The listing builds one solid part. Answer for the finished solid, in the listing's coordinates (mm). Face numbers are marked on the shaded views. A direction names the side the tool comes from. Coordinates: 2 decimals unless noted, no trailing zeros. Order: outer loops, then holes, each group sorted by start corner. A loop starts at its lowest first (then second) coordinate and runs counter-clockwise, first axis right, second up. Notation, with made-up numbers: (-8, 66.25) -> (25, 66.25) arc R21 ccw to (25, 103.25) -> close; hole circle Ø6 at (70, -5). An arc over 180 degrees is marked (long way). Put each result on its own line as item: value. Start each with the question number.
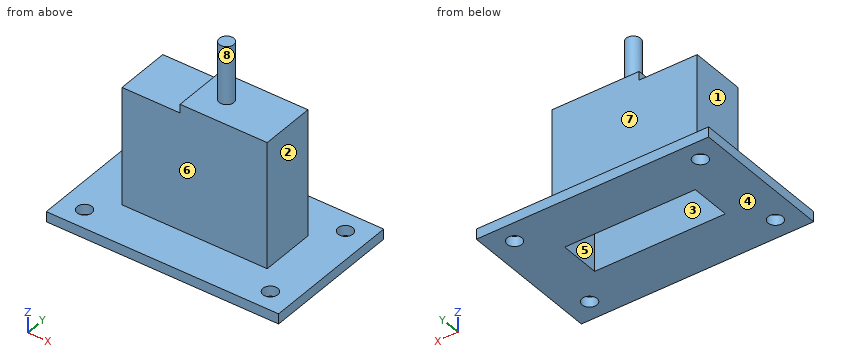
```python
from build123d import *

# Parameters (mm, degrees)
F0_W      = 50
F0_H      = 19
F1_DEPTH  = 44
F2_W      = 30
F2_H      = 19
F3_DEPTH  = 3
F4_R      = 2.5
F5_DEPTH  = 20
F6_W      = 80
F6_H      = 49
F7_DEPTH  = 3.5
F8_R      = 2.55
F9_DEPTH  = 3.5
F10_W     = 45
F10_H     = 14
F11_DEPTH = 42


with BuildPart() as f1:
    # F0 (on Top) → F1 (new body)
    with BuildSketch(Plane.XY):
        Rectangle(F0_W, F0_H)
    extrude(amount=F1_DEPTH)

    # F2 (on face) → F3 (join)
    with BuildSketch(Plane.XY.offset(44)):
        with Locations((10, 0)):
            Rectangle(F2_W, F2_H)
    extrude(amount=F3_DEPTH)

    # F4 (on face) → F5 (join)
    with BuildSketch(Plane.XY.offset(47)):
        with Locations((4, 0)):
            Circle(F4_R)
    extrude(amount=F5_DEPTH)

    # F6 (on face) → F7 (join)
    with BuildSketch(Plane(origin=(0, 0, 0), x_dir=(1, 0, 0), z_dir=(0, 0, -1))):
        Rectangle(F6_W, F6_H)
    extrude(amount=-F7_DEPTH)

    # F8 (on face) → F9 (cut, through all)
    with BuildSketch(Plane.XY.offset(3.5)):
        with Locations((-32, 17.5)):
            Circle(F8_R)
        with Locations((32, 17.5)):
            Circle(F8_R)
        with Locations((-32, -17.5)):
            Circle(F8_R)
        with Locations((32, -17.5)):
            Circle(F8_R)
    extrude(amount=-F9_DEPTH, mode=Mode.SUBTRACT)

    # F10 (on face) → F11 (cut)
    with BuildSketch(Plane(origin=(0, 0, 0), x_dir=(1, 0, 0), z_dir=(0, 0, -1))):
        Rectangle(F10_W, F10_H)
    extrude(amount=-F11_DEPTH, mode=Mode.SUBTRACT)


solid = f1.part
```
(1) Find the intervals of material crossed by L1, parallel to Y at x = 32, z = 1.15; L2, parallel to Y at x = 16, z = 29.5; L3, parallel to X at y = -2, z = 5, in increasing order.
(2) The part is cut by section B-B on z = 18. Determine the outline of the cut face in (x, y).
(3) The part is cut by section D-D on x = 4. Determine the outline of the cut face in (y, z).
(4) The part is cut by section C-C on x = -32. Determine the outline of the cut face in (y, z).
(5) Each of these flat-tipped pins is pushed along its axis until it touches: P1, Ø6, axis at x = -32, y = -17.5, coming from the +Z side; P2, Ø22, axis at x = 1.5, z = 33, coming from the +Y side; P3, Ø4, axis at x = 10, y = -1.5, coming from the -Z side; P4, Ø4, axis at x = 32, y = -17.5, coming from the -Z side. Where does it stop, or does it pass through?
(6) A tool of negligible diameter and unlimited length cuts with its end or side. For the marked faces 5, 6, 7 and 8, from which of +Z, -Z, +X, -X, +Y, -Y can it reach the whole face along a straight path? Write none if from no direction.
(7) For a pull along X with two mould halves and no side action, classify the marked faces 1, 2, 3 and 4 as released by +X, released by -X, zero draft, split by the parting line, or undercut.
(8) The part is cut by section A-A on y = -17.5. Determine the outline of the cut face in (x, z), plus the area to 3 significant figures.
Worked out:
1. L1: -24.5 to -20.05, -14.95 to 14.95, 20.05 to 24.5
1. L2: -9.5 to -7, 7 to 9.5
1. L3: -25 to -22.5, 22.5 to 25
2. outline: (-25, -9.5) -> (25, -9.5) -> (25, 9.5) -> (-25, 9.5) -> close; hole (-22.5, -7) -> (22.5, -7) -> (22.5, 7) -> (-22.5, 7) -> close
3. outline: (-24.5, 0) -> (-7, 0) -> (-7, 42) -> (7, 42) -> (7, 0) -> (24.5, 0) -> (24.5, 3.5) -> (9.5, 3.5) -> (9.5, 47) -> (2.5, 47) -> (2.5, 67) -> (-2.5, 67) -> (-2.5, 47) -> (-9.5, 47) -> (-9.5, 3.5) -> (-24.5, 3.5) -> close
4. outline: (-24.5, 0) -> (-20.05, 0) -> (-20.05, 3.5) -> (-24.5, 3.5) -> close; (-14.95, 0) -> (14.95, 0) -> (14.95, 3.5) -> (-14.95, 3.5) -> close; (20.05, 0) -> (24.5, 0) -> (24.5, 3.5) -> (20.05, 3.5) -> close
5. P1: z = 3.5
5. P2: y = 9.5
5. P3: z = 42
5. P4: through
6. face 5: -Z
6. face 6: +Z, +X, -X, -Y
6. face 7: +Z, +X, -X, +Y
6. face 8: +Z
7. face 1: released by -X
7. face 2: released by +X
7. face 3: undercut
7. face 4: zero draft
8. outline: (-40, 0) -> (-34.55, 0) -> (-34.55, 3.5) -> (-40, 3.5) -> close; (-29.45, 0) -> (29.45, 0) -> (29.45, 3.5) -> (-29.45, 3.5) -> close; (34.55, 0) -> (40, 0) -> (40, 3.5) -> (34.55, 3.5) -> close
8. area: 244 mm2
